Geometry: final body of the model. Coordinates: model frame, mm. A direction names the side the tool comes from. Give positions to 0.01 mm unless a question says otherwise; leave off trailing zeros. Write each loop counter-clockwise with the first axis right and the second up, starting at its lowest first coordinate (ties: lowest second). Pieces come first, ordered by that corner, then holes.
from build123d import *

# Parameters (mm, degrees)
SKETCH_1_W           = 12.7
SKETCH_1_H           = 6.35
EXTRUDE_1_DEPTH      = 5.08
SKETCH_2_W           = 11.7
SKETCH_2_H           = 5.35
CUT_EXTRUDE_1_DEPTH  = 4.08
SKETCH_3_W           = 2
SKETCH_3_H           = 4.08
CUT_EXTRUDE_2_DEPTH  = 1
EXTRUDE_2_DEPTH      = 2
EXTRUDE_2_DEPTH_BACK = 3.58
SKETCH_4_W           = 0.75
SKETCH_4_H           = 0.75


with BuildPart() as part:
    # 草图1 → 拉伸1 (new body)
    with BuildSketch(Plane(origin=(0, 0, 0), x_dir=(1, 0, 0), z_dir=(0, 1, 0))):
        Rectangle(SKETCH_1_W, SKETCH_1_H)
    extrude(amount=EXTRUDE_1_DEPTH)

    # 草图2 → 切除-拉伸1 (cut)
    with BuildSketch(Plane(origin=(0, 5.08, 0), x_dir=(-1, 0, 0), z_dir=(0, 1, 0))):
        Rectangle(SKETCH_2_W, SKETCH_2_H)
    extrude(amount=-CUT_EXTRUDE_1_DEPTH, mode=Mode.SUBTRACT)

    # 草图3 → 切除-拉伸2 (cut)
    with BuildSketch(Plane.XY.offset(3.175)):
        with Locations((0, 3.04)):
            Rectangle(SKETCH_3_W, SKETCH_3_H)
    extrude(amount=-CUT_EXTRUDE_2_DEPTH, mode=Mode.SUBTRACT)

    # 草图4 → 拉伸2 (add, two sides: drawn at the far end of the back side and taken through both)
    with BuildSketch(Plane.XZ.offset(-EXTRUDE_2_DEPTH_BACK)):
        with Locations((-1.27, 0.635)):
            Rectangle(SKETCH_4_W, SKETCH_4_H)
        with Locations((1.27, 0.635)):
            Rectangle(SKETCH_4_W, SKETCH_4_H)
        with Locations((3.81, 0.635)):
            Rectangle(SKETCH_4_W, SKETCH_4_H)
        with Locations((-3.81, 0.635)):
            Rectangle(SKETCH_4_W, SKETCH_4_H)
    extrude(amount=EXTRUDE_2_DEPTH + EXTRUDE_2_DEPTH_BACK)


solid = part.part
Q1. Section C-C on x = 2.25. Output: boundary loops of the cut face in (y, z) (3 decimals).
Filled sheet:
outline: (0, -3.175) - (5.08, -3.175) - (5.08, -2.675) - (1, -2.675) - (1, 2.675) - (5.08, 2.675) - (5.08, 3.175) - (0, 3.175) - close
Q2. Section D-D on z = -1. Output: boundary loops of the cut face in (x, y), plus the area to 3 significant figures.
Filled sheet:
outline: (-6.35, 0) - (6.35, 0) - (6.35, 5.08) - (5.85, 5.08) - (5.85, 1) - (-5.85, 1) - (-5.85, 5.08) - (-6.35, 5.08) - close
area: 16.8 mm2
Q3. Pin query (flat end, axial travel): P1, Ø1, axis at x = 1.5, z = -2.5, coming from the +Y side; P2, Ø0.6, axis at x = -4, y = -0.5, coming from the -Z side; P3, Ø0.6, axis at x = 4, y = -0.5, coming from the +Z side; P4, Ø1, axis at x = -2.5, z = 1, coming from the -Y side. Return the tip coordinate at first contact, or that it passes through.
Filled sheet:
P1: stops at y = 5.08
P2: stops at z = 0.26
P3: stops at z = 1.01
P4: stops at y = 0
Q4. Access query for faces 4 (the flat face through (-3, 3, 2.675)), 5 (the flat face through (6.35, 3, 0)). Directions: +Z, -Z, +X, -X, +Y, -Y. A direction counts if a zero-diameter tool reaches every point of the face in a straight line with its end or side. Return the directions, or none.
Filled sheet:
face 4: +Y
face 5: +Z, -Z, +X, +Y, -Y
Q5. Section A-A on y = -1. Output: boundary loops of the cut face in (x, z) (3 decimals).
Filled sheet:
outline: (-4.185, 0.26) - (-3.435, 0.26) - (-3.435, 1.01) - (-4.185, 1.01) - close; (-1.645, 0.26) - (-0.895, 0.26) - (-0.895, 1.01) - (-1.645, 1.01) - close; (0.895, 0.26) - (1.645, 0.26) - (1.645, 1.01) - (0.895, 1.01) - close; (3.435, 0.26) - (4.185, 0.26) - (4.185, 1.01) - (3.435, 1.01) - close
Q6. Ray query, line 1 along X through (y, z) = (2.5, 0.5) (3 decimals); line 2 along X through (y, z) = (3.5, 2.75); line 3 along X through (y, z) = (4, 1.5). Return the intervals inside material, ascending.
Filled sheet:
line 1: x = -6.35 to -5.85, -4.185 to -3.435, -1.645 to -0.895, 0.895 to 1.645, 3.435 to 4.185, 5.85 to 6.35
line 2: x = -6.35 to -1, 1 to 6.35
line 3: x = -6.35 to -5.85, 5.85 to 6.35
Q7. Section B-B on y = 3. Output: boundary loops of the cut face in (x, z) (3 decimals).
Filled sheet:
outline: (-6.35, -3.175) - (6.35, -3.175) - (6.35, 3.175) - (1, 3.175) - (1, 2.675) - (5.85, 2.675) - (5.85, -2.675) - (-5.85, -2.675) - (-5.85, 2.675) - (-1, 2.675) - (-1, 3.175) - (-6.35, 3.175) - close; (-4.185, 0.26) - (-3.435, 0.26) - (-3.435, 1.01) - (-4.185, 1.01) - close; (-1.645, 0.26) - (-0.895, 0.26) - (-0.895, 1.01) - (-1.645, 1.01) - close; (0.895, 0.26) - (1.645, 0.26) - (1.645, 1.01) - (0.895, 1.01) - close; (3.435, 0.26) - (4.185, 0.26) - (4.185, 1.01) - (3.435, 1.01) - close
Q8. Pull-direction query (Z, two-part tool) for faces 1 (the flat face through (0, 1, 0)), 2 (the flat face through (0, 3, -3.175)), 3 (the flat face through (0, 0, 0)); classes: released by +Z, released by -Z, zero draft, split by the parting line, or undercut.
Filled sheet:
face 1: undercut
face 2: released by -Z
face 3: zero draft
